```python
from build123d import *

# Parameters (mm, degrees)
BOSS_EXTRUDE1_DEPTH         = 152.4
BOSS_EXTRUDE1_DEPTH_BACK    = 152.4
SKETCH3_W                   = 76.2
SKETCH3_H                   = 76.2
SKETCH3_W_2                 = 69.85
SKETCH3_H_2                 = 69.85
F_5_16_CLEARANCE_HOLE3_D    = 8.4328
F_1_2_CLEARANCE_HOLE1_D     = 13.49248
F_1_2_CLEARANCE_HOLE1_DEPTH = 3.175
F_1_2_CLEARANCE_HOLE1_TIP   = 4.053549943


with BuildPart() as part:
    # Sketch3 → Boss-Extrude1 (new, two sides: drawn at the far end of the back side and taken through both)
    with BuildSketch(Plane.XY.offset(-BOSS_EXTRUDE1_DEPTH_BACK)):
        Rectangle(SKETCH3_W, SKETCH3_H)
        Rectangle(SKETCH3_W_2, SKETCH3_H_2, mode=Mode.SUBTRACT)
    extrude(amount=BOSS_EXTRUDE1_DEPTH + BOSS_EXTRUDE1_DEPTH_BACK)

    # 5/16 Clearance Hole3 (through all)
    with Locations(Plane(origin=(0, -38.1, 0), x_dir=(-1, 0, 0), z_dir=(0, -1, 0))):
        with Locations((20, 50.8), (-20, -50.8), (-20, 50.8), (20, -50.8)):
            Hole(F_5_16_CLEARANCE_HOLE3_D / 2)

    # 1/2 Clearance Hole1
    with Locations(Plane(origin=(0, -38.1, 0), x_dir=(-1, 0, 0), z_dir=(0, -1, 0))):
        with Locations((-20, 50.8), (20, 50.8), (-20, -50.8), (20, -50.8)):
            Hole(F_1_2_CLEARANCE_HOLE1_D / 2, depth=F_1_2_CLEARANCE_HOLE1_DEPTH)
            with Locations((0, 0, -(F_1_2_CLEARANCE_HOLE1_DEPTH + F_1_2_CLEARANCE_HOLE1_TIP / 2))):  # 118° drill point
                Cone(0, F_1_2_CLEARANCE_HOLE1_D / 2, F_1_2_CLEARANCE_HOLE1_TIP, mode=Mode.SUBTRACT)


solid = part.part
```
Part model, mm, in its own coordinate system. A direction names the side the tool comes from. Round coordinates to 2 decimals unless told otherwise and drop trailing zeros. Loops run counter-clockwise (first coordinate to the right, second up) from the corner with the lowest first, then second, coordinate; pieces in that order, holes last. Notation, with made-up numbers: (66, 69) -> (120, 69) arc R22 ccw to (120, 95) -> close; hole circle Ø9 at (57.5, -16.5). An arc over 180 degrees is marked (long way). Use CSV: the item, a comma, the result in double quotes. Start each with the question number.
1) Pull direction Y, two halves, no side cores. Call faces 1 (the cylindrical face through (-24.97, -36.49, -55.36)), 2 (the flat face through (-1, 38.1, -2)), 3 (the flat face through (34.925, 0, -2)), 4 (the flat face through (-1, -38.1, -2)): +Y half, -Y half, draft (parallel to the pull), parting line (faces both ways), or undercut.
2) Drop flat-ended pins along their axis: P1, Ø12, axis at x = 15.5, y = 25, coming from the +Z side; P2, Ø12, axis at x = -20, z = 50.8, coming from the -Y side (3 decimals). Give the stop position or say it passes through.
3) Wall check: L1, parallel to X at y = 36.55, z = 50.8; L2, parallel to Z at x = 20, y = 35; L3, parallel to X at y = -36.65, z = 50.8. Give the ranges that are in metal, low to high. Write a range as [from, to].
4) Which spindle directions (+Z, -Z, +X, -X, +Y, -Y) get a long thin tool onto all of the face, cutting with end or side? Do faces 5 (the cylindrical face through (15.03, -36.49, -55.36)), 6 (the flat face through (0, 34.925, -2)), 7 (the flat face through (-3, -37, 152.4)). Say none if no direction does.
5) Cut at A-A, the plane y = -11. Write the cut outline in (x, z) (3 decimals).
6) Cut at D-D, the plane z = -50.8. Write the cut outline in (x, y) (3 decimals), plus the area to 3 significant figures.
7) Cut at B-B, the plane x = -20. Write the cut outline in (y, z) (3 decimals), plus the area to 3 significant figures.
Determined:
1,face 1,"draft"
1,face 2,"+Y half"
1,face 3,"undercut"
1,face 4,"-Y half"
2,P1,"passes through"
2,P2,"stops at y = 34.925"
3,L1,"x = [-38.1, -24.22], [-15.78, 15.78], [24.22, 38.1]"
3,L2,"z = [-152.4, -55.02], [-46.58, 46.58], [55.02, 152.4]"
3,L3,"x = [-38.1, -26.75], [-13.25, 13.25], [26.75, 38.1]"
4,face 5,"-Y"
4,face 6,"+Z, -Z"
4,face 7,"+Z, +X, -X, +Y, -Y"
5,outline,"(-38.1, -152.4) -> (-34.925, -152.4) -> (-34.925, 152.4) -> (-38.1, 152.4) -> close; (34.925, -152.4) -> (38.1, -152.4) -> (38.1, 152.4) -> (34.925, 152.4) -> close"
6,outline,"(-38.1, -38.1) -> (-26.746, -38.1) -> (-26.746, -34.925) -> (-34.925, -34.925) -> (-34.925, 34.925) -> (-24.216, 34.925) -> (-24.216, 38.1) -> (-38.1, 38.1) -> close; (-15.784, 34.925) -> (15.784, 34.925) -> (15.784, 38.1) -> (-15.784, 38.1) -> close; (-13.254, -38.1) -> (13.254, -38.1) -> (13.254, -34.925) -> (-13.254, -34.925) -> close; (24.216, 34.925) -> (34.925, 34.925) -> (34.925, -34.925) -> (26.746, -34.925) -> (26.746, -38.1) -> (38.1, -38.1) -> (38.1, 38.1) -> (24.216, 38.1) -> close"
6,area,"788 mm2"
7,outline,"(-38.1, -152.4) -> (-34.925, -152.4) -> (-34.925, -57.546) -> (-38.1, -57.546) -> close; (-38.1, -44.054) -> (-34.925, -44.054) -> (-34.925, 44.054) -> (-38.1, 44.054) -> close; (-38.1, 57.546) -> (-34.925, 57.546) -> (-34.925, 152.4) -> (-38.1, 152.4) -> close; (34.925, -152.4) -> (38.1, -152.4) -> (38.1, -55.016) -> (34.925, -55.016) -> close; (34.925, -46.584) -> (38.1, -46.584) -> (38.1, 46.584) -> (34.925, 46.584) -> close; (34.925, 55.016) -> (38.1, 55.016) -> (38.1, 152.4) -> (34.925, 152.4) -> close"
7,area,"1,800 mm2"
